Build history of the part. All positions in model axes, mm. Face numbers are marked on the shaded views. A direction names the side the tool comes from. Give positions to 0.01 mm unless a question says otherwise; leave off trailing zeros. Loops run counter-clockwise (first coordinate to the right, second up) from the corner with the lowest first, then second, coordinate; pieces in that order, holes last. Notation, with made-up numbers: (89, -30) -> (122, -30) arc R4 cw to (122, -24) -> close; hole circle Ø3 at (-16.75, 72). An arc over 180 degrees is marked (long way). Answer in a Markdown table with one row per item. Add a question column.
Autodesk Inventor part; units mm, degrees
ref_plane "YZ Plane" through (0, 0, 0) normal (1, 0, 0) x (0, 1, 0)
ref_plane "XZ Plane" through (0, 0, 0) normal (0, 1, 0) x (-1, 0, 0)
ref_plane "XY Plane" through (0, 0, 0) normal (0, 0, 1) x (1, 0, 0)
sketch "Sketch_1" plane through (0, 0, 0) normal (0, 0, 1) x (1, 0, 0)
  line L0 (8, 0) -> (0, 0)
  line L1 (0, 0) -> (0, 2.75)
  line L2 (0, 2.75) -> (0.1072, 3.15)
  line L3 (0.1072, 3.15) -> (7.8928, 3.15)
  line L4 (7.8928, 3.15) -> (8, 2.75)
  line L5 (8, 2.75) -> (8, 0)
  line L6 (8, 0) -> (0, 0)
revolve "Revolution1" add sketch "Sketch_1" angle 360 about axis through (8, 0, 0) along (1, 0, 0)
sketch "Sketch_5" plane through (0, 0, 0) normal (0, 0, 1) x (1, 0, 0)
  line L0 (0, 0) -> (-6, 0)
  line L1 (-6, 0) -> (-6, 1.1935)
  line L2 (-6, 1.1935) -> (-5.6935, 1.5)
  line L3 (-5.6935, 1.5) -> (-0.6, 1.5)
  line L4 (-0.6, 1.5) -> (-0.6, 1.2295)
  line L5 (-0.6, 1.2295) -> (0, 1.2295)
  line L6 (0, 1.2295) -> (0, 0)
  line L7 (0, 0) -> (-6, 0)
revolve "Revolution2" add sketch "Sketch_5" angle 360 about axis through (0, 0, 0) along (1, 0, 0)
thread "Thread1"
sketch "Sketch_6" plane through (0, 0, 0) normal (1, 0, 0) x (0, 1, 0)
  circle A0 centre (0, 0) radius 6.3
  line L0 (1.5877, 2.75) -> (-1.5877, 2.75)
  line L1 (-1.5877, 2.75) -> (-3.1754, 0)
  line L2 (-3.1754, 0) -> (-1.5877, -2.75)
  line L3 (-1.5877, -2.75) -> (1.5877, -2.75)
  line L4 (1.5877, -2.75) -> (3.1754, 0)
  line L5 (3.1754, 0) -> (1.5877, 2.75)
extrude "Extrusion1" cut sketch "Sketch_6" along normal blind 8
sketch "Sketch4" plane through (8, 0, 0) normal (1, 0, 0) x (0, 0, -1)
  point P0 (0, 0)
hole "Hole1" at (8, 0, 0) direction (-1, 0, 0) diameter 2.459 depth 6.4901 tip angle 120 countersink diameter 3 countersink angle 90
sketch "スケッチ5" plane through (-6, 0, 0) normal (-1, 0, 0) x (0, 0, 1)
  circle A0 centre (0, 0) radius 1.1935
  circle A1 centre (0, 0) radius 1.2
  circle A2 centre (0, 0) radius 2.2848
  dimension "d13" = 2.4
extrude "押し出し2" cut sketch "スケッチ5" against normal blind 6 contours A2
sketch "スケッチ6" plane through (-6, 0, 0) normal (-1, 0, 0) x (0, 0, 1)
  circle A0 centre (0, 0) radius 1.1935
  circle A1 centre (0, 0) radius 1.9337
extrude "押し出し3" cut sketch "スケッチ6" against normal blind 3 contours A0 | A1
properties part number "SLCG5.5-8" material "ステンレス鋼 AISI 302"
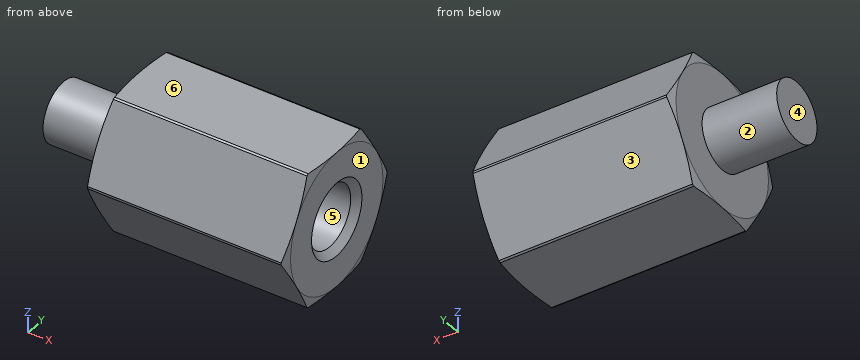
(1) Wall check: line 1 along Z through (x, y) = (3.5, 0); line 2 along Y through (x, z) = (3.75, 0); line 3 along X through (y, z) = (0, -2.5). Give the ranges that are in metal, low to high. Write a range as from..to.
(2) Saw through at B-B, the plane x = 0.5. List the corners of the cut face in (y, z), then the cut area to 3 significant figures.
(3) Two-plate mould, pull along Z, no slides. Class the marked faces 3, 4, 5 and 6: released by +Z, released by -Z, zero draft, split by the parting line, or undercut.
(4) Flat gauge pin, fed straight in: pin 1 Ø2 at (x, z) = (0, -1.5) entering from -Y. Where does the tip first touch, or does it go through?
(5) Saw through at A-A, the plane x = 4.25. List the corners of the cut face in (y, z).
(6) 3-axis set-ups, long thin cutter, end or side, ignore diameter. For the marked faces 1 and 2: which of +Z, -Z, +X, -X, +Y, -Y reach the whole face in a straight line?
Worked answers:
| question | item | result |
|---|---|---|
| 1 | line 1 | -2.75..-1.23, 1.23..2.75 |
| 1 | line 2 | -3.15..-1.23, 1.23..3.15 |
| 1 | line 3 | 0..8 |
| 2 | outline | (-3.15, -0.04) -> (-1.61, -2.71) arc R3.15 ccw to (-1.54, -2.75) -> (1.54, -2.75) arc R3.15 ccw to (1.61, -2.71) -> (3.15, -0.04) arc R3.15 ccw to (3.15, 0.04) -> (1.61, 2.71) arc R3.15 ccw to (1.54, 2.75) -> (-1.54, 2.75) arc R3.15 ccw to (-1.61, 2.71) -> (-3.15, 0.04) arc R3.15 ccw to start |
| 2 | area | 26.2 mm^2 |
| 3 | face 3 | released by -Z |
| 3 | face 4 | zero draft |
| 3 | face 5 | undercut |
| 3 | face 6 | released by +Z |
| 4 | pin 1 | y = -2.89 |
| 5 | outline | (-3.15, -0.04) -> (-1.61, -2.71) arc R3.15 ccw to (-1.54, -2.75) -> (1.54, -2.75) arc R3.15 ccw to (1.61, -2.71) -> (3.15, -0.04) arc R3.15 ccw to (3.15, 0.04) -> (1.61, 2.71) arc R3.15 ccw to (1.54, 2.75) -> (-1.54, 2.75) arc R3.15 ccw to (-1.61, 2.71) -> (-3.15, 0.04) arc R3.15 ccw to start; hole circle Ø2.46 at (0, 0) |
| 6 | face 1 | +Z, -Z, +X, +Y, -Y |
| 6 | face 2 | -X |
